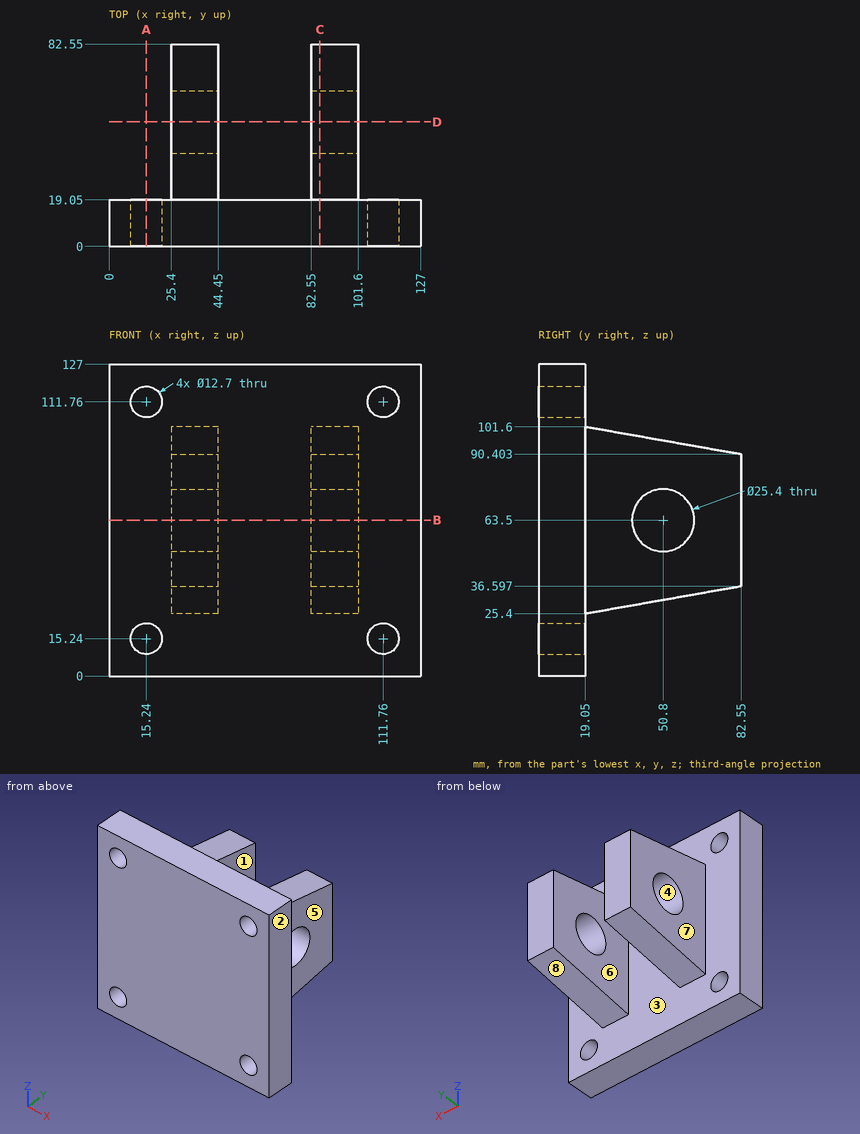
The drawing under review shows one solid part. Ordinate dimensions are in mm from its lowest x, y, z. A direction names the side the tool comes from. Round coordinates to 2 decimals unless told otherwise and drop trailing zeros. Loops run counter-clockwise (first coordinate to the right, second up) from the corner with the lowest first, then second, coordinate; pieces in that order, holes last. Notation, with made-up numbers: (-13, -13) - (25, -13) arc R16 ccw to (25, 10) - close; hole circle Ø11 at (13, -18). An arc over 180 degrees is marked (long way). One line per item, written item: value. Start each with the question number.
1) Consider section D-D on y = 50.8. Give the boundary of the cut face in (x, z).
2) To check wall thickness, follow L1, parallel to Z at x = 15.24, y = 11; L2, parallel to X at y = 55, z = 84; L3, parallel to Z at x = 107.5, y = 17.5. State the ranges of each line that lie inside material, in increasing order. Write a range as from..to.
3) Draft analysis for pull direction X (two halves, no side actions). For the marked faces 1, 2, 3 and 4, state which applies: +X half, -X half, draft (parallel to the pull), parting line (faces both ways), or undercut.
4) For the marked faces 5, 6, 7 and 8, list the 3-axis set-ups (+Z, -Z, +X, -X, +Y, -Y) from which the entire face can be reached by the end or side of a thin tool; tool diameter is ignored.
5) Consider section C-C on x = 86. Give the boundary of the cut face in (y, z), then the cut area to 3 significant figures.
6) Insertion check: pin 1 Ø1.5 at (y, z) = (34, 54) entering from +X; pin 2 Ø6 at (x, y) = (81, 42.5) entering from -Z; pin 3 Ø1.5 at (x, y) = (45, 48) entering from -Z (1 decimal). Each pin has a flat end and moves straight along its axis. Give the tip position at first contact, or say it passes through.
7) Consider section A-A on x = 15.24. Give the boundary of the cut face in (y, z), then the cut area to 3 significant figures.
8) Consider section B-B on z = 63.5. Give the boundary of the cut face in (x, y).
Reported:
1. outline: (25.4, 31) - (44.45, 31) - (44.45, 50.8) - (25.4, 50.8) - close; (25.4, 76.2) - (44.45, 76.2) - (44.45, 96) - (25.4, 96) - close; (82.55, 31) - (101.6, 31) - (101.6, 50.8) - (82.55, 50.8) - close; (82.55, 76.2) - (101.6, 76.2) - (101.6, 96) - (82.55, 96) - close
2. L1: z = 0..8.89, 21.59..105.41, 118.11..127
2. L2: x = 25.4..44.45, 82.55..101.6
2. L3: z = 0..10.53, 19.95..107.05, 116.47..127
3. face 1: undercut
3. face 2: +X half
3. face 3: undercut
3. face 4: draft
4. face 5: +Z, -Z, +X, +Y
4. face 6: +Z, -Z, +Y
4. face 7: +Z, -Z, -X, +Y
4. face 8: -Z, +X, -X, +Y
5. outline: (0, 0) - (19.05, 0) - (19.05, 25.4) - (82.55, 36.6) - (82.55, 90.4) - (19.05, 101.6) - (19.05, 127) - (0, 127) - close; hole circle Ø25.4 at (50.8, 63.5)
5. area: 6,040 mm^2
6. pin 1: stops at x = 101.6
6. pin 2: stops at z = 29.08
6. pin 3: stops at z = 30.4
7. outline: (0, 0) - (19.05, 0) - (19.05, 8.89) - (0, 8.89) - close; (0, 21.59) - (19.05, 21.59) - (19.05, 105.41) - (0, 105.41) - close; (0, 118.11) - (19.05, 118.11) - (19.05, 127) - (0, 127) - close
7. area: 1,940 mm^2
8. outline: (0, 0) - (127, 0) - (127, 19.05) - (101.6, 19.05) - (101.6, 38.1) - (82.55, 38.1) - (82.55, 19.05) - (44.45, 19.05) - (44.45, 38.1) - (25.4, 38.1) - (25.4, 19.05) - (0, 19.05) - close; (25.4, 63.5) - (44.45, 63.5) - (44.45, 82.55) - (25.4, 82.55) - close; (82.55, 63.5) - (101.6, 63.5) - (101.6, 82.55) - (82.55, 82.55) - close
